Autodesk Inventor part; units mm, degrees
ref_plane "YZ Plane" through (0, 0, 0) normal (1, 0, 0) x (0, 1, 0)
ref_plane "XZ Plane" through (0, 0, 0) normal (0, 1, 0) x (-1, 0, 0)
ref_plane "XY Plane" through (0, 0, 0) normal (0, 0, 1) x (1, 0, 0)
sketch "Sketch1" plane through (0, 0, 0) normal (0, 0, 1) x (1, 0, 0)
  circle A0 centre (0, 0) radius 9
  circle A1 centre (0, 0) radius 4.5
  dimension "d0" = 18
  dimension "d1" = 9
extrude "Extrusion1" add sketch "Sketch1" along normal blind 55 contours A0 | A1
sketch "Sketch2" plane through (0, 0, 55) normal (0, 0, 1) x (1, 0, 0)
  circle A0 centre (0, 0) radius 4.5
  dimension "d4" = 9
extrude "Extrusion2" add sketch "Sketch2" along normal blind 10
fillet "Fillet1" radius 6.7625 1 edges at (-9, 0, 55)
fillet "Fillet2" radius 2 1 edges at (-4.5, 0, 65)
fillet "Fillet3" radius 5.175 1 edges at (-9, 0, 0)
properties part number "8g_CO2_Cylinder"
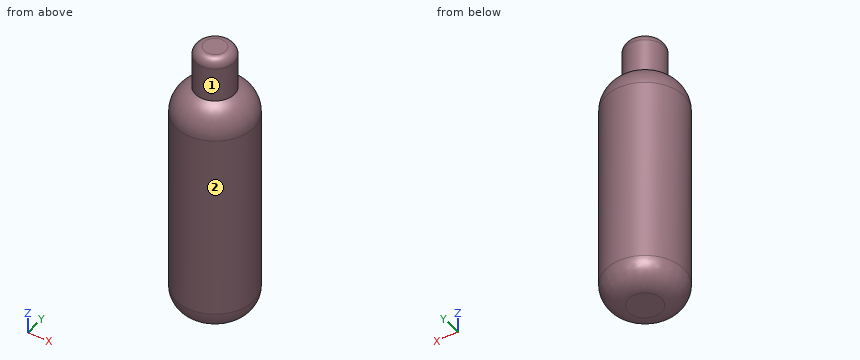
Source: CAD feature listing. Evaluate the final solid. Frame: model axes, mm. Face numbers are marked on the shaded views. A direction names the side the tool comes from. Coordinates: 2 decimals unless noted, no trailing zeros. Write each loop counter-clockwise with the first axis right and the second up, starting at its lowest first coordinate (ties: lowest second). Pieces come first, ordered by that corner, then holes. Notation, with made-up numbers: M 2.25,-23.5 L 34.25,-23.5 A29 ccw 34.25,9.5 Z; hole C -12.75,67 d2. An arc over 180 degrees is marked long. Answer as a JSON object with one key per item and string values.
1. Access query for the marked faces 1 and 2. Directions: +Z, -Z, +X, -X, +Y, -Y. A direction counts if a zero-diameter tool reaches every point of the face in a straight line with its end or side. Return the directions, or none.
Evaluation:
{"face 1": "+Z", "face 2": "+Z, -Z"}
2. Ray query, L1, parallel to Z at x = 2.5, y = 0.75; L2, parallel to X at y = -1.25, z = 16.5; L3, parallel to Z at x = -3.5, y = -5.5. Return the intervals inside material, ascending.
Evaluation:
{"L1": "0 to 65", "L2": "-8.91 to 8.91", "L3": "0.76 to 53.86"}
3. Cut plane A-A on z = 25. Output: boundary loops of the cut face in (x, y), plus the area to 3 significant figures.
Evaluation:
{"outline": "C 0,0 d18", "area": "254 mm^2"}
4. Contact query for flat-ended pins moving along their axis: P1, Ø4, axis at y = 4, z = 43, coming from the +X side; P2, Ø8, axis at x = 0.5, y = -3.5, coming from the -Z side; P3, Ø1.5, axis at x = 2, z = 13.5, coming from the -Y side; P4, Ø5, axis at x = -5, z = 10.5, coming from the -Y side. Output: stop coordinate, or through.
Evaluation:
{"P1": "x = 8.77", "P2": "z = 0", "P3": "y = -8.91", "P4": "y = -8.65"}
